Work out the finished part from the listing and answer in its coordinate system (mm). Give positions to 0.01 mm unless a question says otherwise; leave off trailing zeros. Write each loop counter-clockwise with the first axis right and the second up, starting at its lowest first coordinate (ties: lowest second). Pieces come first, ordered by that corner, then holes. Notation, with made-up numbers: (75, 77.5) -> (123, 77.5) arc R22 cw to (123, 110.5) -> close; hole circle Ø7 at (8, 1.25). An arc over 180 degrees is marked (long way). Use a Markdown table: item, result. Add a question column.
Q1. Section C-C, the plane z = 2.7 is taken. Give the vertices of the cut face in (x, y), plus the area to 3 significant figures.
Q2. Consider line 1 (Y direction, x = -25, z = 1.1); line 2 (X direction, y = -9.75, z = 3.65); line 3 (Y direction, x = 0, z = 3). Determine where each line is inside the solid, lowest interval first.
Q3. Section B-B, the plane y = -10 is taken. Give the vertices of the cut face in (x, z), plus the area to 3 significant figures.
Q4. For a pull along Y with two mould halves and no side action, classify faces 1 (the face through (23.35, -9.93, 2.46)), 2 (the face through (30, -10, 2)), 3 (the face through (29, -2, 2)) as pulls with the +Y half, pulls with the -Y half, needs draft (parallel to the pull), parting line crosses it, or undercut.
Q5. This flat-tipped pin is pushed along its axis until it touches: pin 1 Ø3 at (x, y) = (-10, -9) entering from -Z. Where does it stop, or does it pass through?
Q6. Section A-A, the plane x = 0 is taken. Give the vertices of the cut face in (y, z).
from build123d import *

# Parameters (mm, degrees)
ESQUISSE1_W        = 60
ESQUISSE1_H        = 20
ESQUISSE1_R        = 2.25
ESQUISSE1_R_2      = 1.65
BOSS_EXTRU_1_DEPTH = 5
CONG_1_R           = 1
CONG_3_R           = 5


with BuildPart() as part:
    # Esquisse1 → Boss.-Extru.1 (new body)
    with BuildSketch(Plane.XY):
        with Locations((0, -10)):
            Rectangle(ESQUISSE1_W, ESQUISSE1_H)
        with Locations((0, -10)):
            Circle(ESQUISSE1_R, mode=Mode.SUBTRACT)
        with Locations((25, -10)):
            Circle(ESQUISSE1_R_2, mode=Mode.SUBTRACT)
        with Locations((-25, -10)):
            Circle(ESQUISSE1_R_2, mode=Mode.SUBTRACT)
    extrude(amount=BOSS_EXTRU_1_DEPTH)

    # Congé1
    cong_1_edges = [part.edges().sort_by_distance(p)[0] for p in [
        (-30, -10, 5),
        (0, -20, 5),
        (30, -10, 5),
        (0, 0, 5),
    ]]
    fillet(cong_1_edges, radius=CONG_1_R)

    # Congé3
    # the kernel refuses this fillet: 5 mm, written as the material it takes off along each edge
    with BuildSketch(Plane(origin=(-25, -5, 5), x_dir=(0, 1, 0), z_dir=(1, 0, 0))) as cong_3_piece_1:
        with BuildLine():
            CenterArc((4, -1), 1, 0, 90)
            Line((5, -1), (5, 0))
            Line((5, 0), (4, 0))
        make_face()
    revolve(axis=Axis((-25, -5, 5), (0, 0, 1)), revolution_arc=90, mode=Mode.SUBTRACT)
    with BuildSketch(Plane(origin=(25, -5, 5), x_dir=(1, 0, 0), z_dir=(0, -1, 0))) as cong_3_piece_2:
        with BuildLine():
            CenterArc((4, -1), 1, 0, 90)
            Line((5, -1), (5, 0))
            Line((5, 0), (4, 0))
        make_face()
    revolve(axis=Axis((25, -5, 5), (0, 0, 1)), revolution_arc=90, mode=Mode.SUBTRACT)
    with BuildSketch(Plane(origin=(-25, -15, 5), x_dir=(-1, 0, 0), z_dir=(0, 1, 0))) as cong_3_piece_3:
        with BuildLine():
            CenterArc((4, -1), 1, 0, 90)
            Line((5, -1), (5, 0))
            Line((5, 0), (4, 0))
        make_face()
    revolve(axis=Axis((-25, -15, 5), (0, 0, 1)), revolution_arc=90, mode=Mode.SUBTRACT)
    with BuildSketch(Plane(origin=(25, -15, 5), x_dir=(0, -1, 0), z_dir=(-1, 0, 0))) as cong_3_piece_4:
        with BuildLine():
            CenterArc((4, -1), 1, 0, 90)
            Line((5, -1), (5, 0))
            Line((5, 0), (4, 0))
        make_face()
    revolve(axis=Axis((25, -15, 5), (0, 0, 1)), revolution_arc=90, mode=Mode.SUBTRACT)
    with BuildSketch(Plane(origin=(30, -20, -12.5), x_dir=(0, 1, 0), z_dir=(0, 0, 1)), Plane(origin=(30, 0, -12.5), x_dir=(-1, 0, 0), z_dir=(0, 0, 1))) as cong_3_piece_5:
        with BuildLine():
            CenterArc((CONG_3_R, CONG_3_R), CONG_3_R, 180, 90)
            Line((0, CONG_3_R), (0, 0))
            Line((0, 0), (CONG_3_R, 0))
        make_face()
    extrude(amount=17.5, mode=Mode.SUBTRACT)
    with BuildSketch(Plane(origin=(-30, -20, -12.5), x_dir=(0, 1, 0), z_dir=(0, 0, 1)), Plane(origin=(-30, 0, -12.5), x_dir=(1, 0, 0), z_dir=(0, 0, 1))) as cong_3_piece_6:
        with BuildLine():
            CenterArc((CONG_3_R, -CONG_3_R), CONG_3_R, 90, 90)
            Line((0, -CONG_3_R), (0, 0))
            Line((0, 0), (CONG_3_R, 0))
        make_face()
    extrude(amount=17.5, mode=Mode.SUBTRACT)


solid = part.part
Result set:
| question | item | result |
|---|---|---|
| 1 | outline | (-30, -15) arc R5 ccw to (-25, -20) -> (25, -20) arc R5 ccw to (30, -15) -> (30, -5) arc R5 ccw to (25, 0) -> (-25, 0) arc R5 ccw to (-30, -5) -> close; hole circle Ø3.3 at (-25, -10); hole circle Ø4.5 at (0, -10); hole circle Ø3.3 at (25, -10) |
| 1 | area | 1,150 mm2 |
| 2 | line 1 | y = -20 to -11.65, -8.35 to 0 |
| 2 | line 2 | x = -30 to -26.63, -23.37 to -2.24, 2.24 to 23.37, 26.63 to 30 |
| 2 | line 3 | y = -20 to -12.25, -7.75 to 0 |
| 3 | outline | (-30, 0) -> (-26.65, 0) -> (-26.65, 5) -> (-29, 5) arc R1 ccw to (-30, 4) -> close; (-23.35, 0) -> (-2.25, 0) -> (-2.25, 5) -> (-23.35, 5) -> close; (2.25, 0) -> (23.35, 0) -> (23.35, 5) -> (2.25, 5) -> close; (26.65, 0) -> (30, 0) -> (30, 4) arc R1 ccw to (29, 5) -> (26.65, 5) -> close |
| 3 | area | 244 mm2 |
| 4 | face 1 | undercut |
| 4 | face 2 | needs draft |
| 4 | face 3 | pulls with the +Y half |
| 5 | pin 1 | stops at z = 0 |
| 6 | outline | (-20, 0) -> (-12.25, 0) -> (-12.25, 5) -> (-19, 5) arc R1 ccw to (-20, 4) -> close; (-7.75, 0) -> (0, 0) -> (0, 4) arc R1 ccw to (-1, 5) -> (-7.75, 5) -> close |
